from build123d import *

# Parameters (mm, degrees)
DODANIE_WYCI_GNI_CIE1_DEPTH = 5.325088567


with BuildPart() as part:
    # Szkic1 → Dodanie-wyciągnięcie1 (new body)
    with BuildSketch(Plane.XY):
        with BuildLine():
            Line((-0.951045555, 20.39370068), (-1.925922284, 17.39370068))
            ThreePointArc((-1.925922284, 17.39370068), (-2.737603138, 17.28454596), (-3.543288168, 17.13753509))
            Line((-3.543288168, 17.13753509), (-5.397502016, 19.689451162))
            ThreePointArc((-5.397502016, 19.689451162), (-6.515515156, 20.052693732), (-7.206498161, 19.101672684))
            Line((-7.206498161, 19.101672684), (-7.206610043, 15.947249659))
            ThreePointArc((-7.206610043, 15.947249659), (-7.944833745, 15.592614173), (-8.665656885, 15.203828161))
            Line((-8.665656885, 15.203828161), (-11.217704483, 17.05786098))
            ThreePointArc((-11.217704483, 17.05786098), (-12.393246293, 17.057840133), (-12.756528516, 15.939839877))
            Line((-12.756528516, 15.939839877), (-11.7818646, 12.93977073))
            ThreePointArc((-11.7818646, 12.93977073), (-12.374368671, 12.374368671), (-12.93977073, 11.7818646))
            Line((-12.93977073, 11.7818646), (-15.939839877, 12.756528516))
            ThreePointArc((-15.939839877, 12.756528516), (-17.057840133, 12.393246293), (-17.05786098, 11.217704483))
            Line((-17.05786098, 11.217704483), (-15.203828161, 8.665656885))
            ThreePointArc((-15.203828161, 8.665656885), (-15.592614173, 7.944833745), (-15.947249659, 7.206610043))
            Line((-15.947249659, 7.206610043), (-19.101672684, 7.206498161))
            ThreePointArc((-19.101672684, 7.206498161), (-20.052693732, 6.515515156), (-19.689451162, 5.397502016))
            Line((-19.689451162, 5.397502016), (-17.13753509, 3.543288168))
            ThreePointArc((-17.13753509, 3.543288168), (-17.28454596, 2.737603138), (-17.39370068, 1.925922284))
            Line((-17.39370068, 1.925922284), (-20.39370068, 0.951045555))
            ThreePointArc((-20.39370068, 0.951045555), (-21.084649954, 0), (-20.39370068, -0.951045555))
            Line((-20.39370068, -0.951045555), (-17.39370068, -1.925922284))
            ThreePointArc((-17.39370068, -1.925922284), (-17.28454596, -2.737603138), (-17.13753509, -3.543288168))
            Line((-17.13753509, -3.543288168), (-19.689451162, -5.397502016))
            ThreePointArc((-19.689451162, -5.397502016), (-20.052693732, -6.515515156), (-19.101672684, -7.206498161))
            Line((-19.101672684, -7.206498161), (-15.947249659, -7.206610043))
            ThreePointArc((-15.947249659, -7.206610043), (-15.592614173, -7.944833745), (-15.203828161, -8.665656885))
            Line((-15.203828161, -8.665656885), (-17.05786098, -11.217704483))
            ThreePointArc((-17.05786098, -11.217704483), (-17.057840133, -12.393246293), (-15.939839877, -12.756528516))
            Line((-15.939839877, -12.756528516), (-12.93977073, -11.7818646))
            ThreePointArc((-12.93977073, -11.7818646), (-12.374368671, -12.374368671), (-11.7818646, -12.93977073))
            Line((-11.7818646, -12.93977073), (-12.756528516, -15.939839877))
            ThreePointArc((-12.756528516, -15.939839877), (-12.393246293, -17.057840133), (-11.217704483, -17.05786098))
            Line((-11.217704483, -17.05786098), (-8.665656885, -15.203828161))
            ThreePointArc((-8.665656885, -15.203828161), (-7.944833745, -15.592614173), (-7.206610043, -15.947249659))
            Line((-7.206610043, -15.947249659), (-7.206498161, -19.101672684))
            ThreePointArc((-7.206498161, -19.101672684), (-6.515515156, -20.052693732), (-5.397502016, -19.689451162))
            Line((-5.397502016, -19.689451162), (-3.543288168, -17.13753509))
            ThreePointArc((-3.543288168, -17.13753509), (-2.737603138, -17.28454596), (-1.925922284, -17.39370068))
            Line((-1.925922284, -17.39370068), (-0.951045555, -20.39370068))
            ThreePointArc((-0.951045555, -20.39370068), (0, -21.084649954), (0.951045555, -20.39370068))
            Line((0.951045555, -20.39370068), (1.925922284, -17.39370068))
            ThreePointArc((1.925922284, -17.39370068), (2.737603138, -17.28454596), (3.543288168, -17.13753509))
            Line((3.543288168, -17.13753509), (5.397502016, -19.689451162))
            ThreePointArc((5.397502016, -19.689451162), (6.515515156, -20.052693732), (7.206498161, -19.101672684))
            Line((7.206498161, -19.101672684), (7.206610043, -15.947249659))
            ThreePointArc((7.206610043, -15.947249659), (7.944833745, -15.592614173), (8.665656885, -15.203828161))
            Line((8.665656885, -15.203828161), (11.217704483, -17.05786098))
            ThreePointArc((11.217704483, -17.05786098), (12.393246293, -17.057840133), (12.756528516, -15.939839877))
            Line((12.756528516, -15.939839877), (11.7818646, -12.93977073))
            ThreePointArc((11.7818646, -12.93977073), (12.374368671, -12.374368671), (12.93977073, -11.7818646))
            Line((12.93977073, -11.7818646), (15.939839877, -12.756528516))
            ThreePointArc((15.939839877, -12.756528516), (17.057840133, -12.393246293), (17.05786098, -11.217704483))
            Line((17.05786098, -11.217704483), (15.203828161, -8.665656885))
            ThreePointArc((15.203828161, -8.665656885), (15.592614173, -7.944833745), (15.947249659, -7.206610043))
            Line((15.947249659, -7.206610043), (19.101672684, -7.206498161))
            ThreePointArc((19.101672684, -7.206498161), (20.052693732, -6.515515156), (19.689451162, -5.397502016))
            Line((19.689451162, -5.397502016), (17.13753509, -3.543288168))
            ThreePointArc((17.13753509, -3.543288168), (17.28454596, -2.737603138), (17.39370068, -1.925922284))
            Line((17.39370068, -1.925922284), (20.39370068, -0.951045555))
            ThreePointArc((20.39370068, -0.951045555), (21.084649954, 0), (20.39370068, 0.951045555))
            Line((20.39370068, 0.951045555), (17.39370068, 1.925922284))
            ThreePointArc((17.39370068, 1.925922284), (17.28454596, 2.737603138), (17.13753509, 3.543288168))
            Line((17.13753509, 3.543288168), (19.689451162, 5.397502016))
            ThreePointArc((19.689451162, 5.397502016), (20.052693732, 6.515515156), (19.101672684, 7.206498161))
            Line((19.101672684, 7.206498161), (15.947249659, 7.206610043))
            ThreePointArc((15.947249659, 7.206610043), (15.592614173, 7.944833745), (15.203828161, 8.665656885))
            Line((15.203828161, 8.665656885), (17.05786098, 11.217704483))
            ThreePointArc((17.05786098, 11.217704483), (17.057840133, 12.393246293), (15.939839877, 12.756528516))
            Line((15.939839877, 12.756528516), (12.93977073, 11.7818646))
            ThreePointArc((12.93977073, 11.7818646), (12.374368671, 12.374368671), (11.7818646, 12.93977073))
            Line((11.7818646, 12.93977073), (12.756528516, 15.939839877))
            ThreePointArc((12.756528516, 15.939839877), (12.393246293, 17.057840133), (11.217704483, 17.05786098))
            Line((11.217704483, 17.05786098), (8.665656885, 15.203828161))
            ThreePointArc((8.665656885, 15.203828161), (7.944833745, 15.592614173), (7.206610043, 15.947249659))
            Line((7.206610043, 15.947249659), (7.206498161, 19.101672684))
            ThreePointArc((7.206498161, 19.101672684), (6.515515156, 20.052693732), (5.397502016, 19.689451162))
            Line((5.397502016, 19.689451162), (3.543288168, 17.13753509))
            ThreePointArc((3.543288168, 17.13753509), (2.737603138, 17.28454596), (1.925922284, 17.39370068))
            Line((1.925922284, 17.39370068), (0.951045555, 20.39370068))
            ThreePointArc((0.951045555, 20.39370068), (0, 21.084649954), (-0.951045555, 20.39370068))
        make_face()
        with BuildLine():
            Line((-2, 1.5), (-2, -1.5))
            ThreePointArc((-2, -1.5), (2.5, 0), (-2, 1.5))
        make_face(mode=Mode.SUBTRACT)
    extrude(amount=DODANIE_WYCI_GNI_CIE1_DEPTH)


solid = part.part
CAD build for the part. Positions are in the model's coordinates, mm. A direction names the side the tool comes from. Coordinates: 2 decimals unless noted, no trailing zeros. Write each loop counter-clockwise with the first axis right and the second up, starting at its lowest first coordinate (ties: lowest second). Pieces come first, ordered by that corner, then holes. Notation, with made-up numbers: (3, 87) - (29, 87) arc R20 ccw to (29, 126) - close; hole circle Ø1 at (45, 34.5). An arc over 180 degrees is marked (long way). Use a Markdown table: item, result. Add a question column.
Item 1: Band-saw the part on B-B, the plane y = 0. Give the cut face in (x, z), and give its area (3 significant figures).
Item 2: Band-saw the part on A-A, the plane x = 0. Give the cut face in (y, z), and give its area (3 significant figures).
Item 3: Band-saw the part on D-D, the plane x = -13.5. Give the cut face in (y, z), and give its area (3 significant figures).
Item 4: Drill centre lines: L1, parallel to X at y = 19.5, z = 2.1; L2, parallel to Y at x = -16, z = 3.35; L3, parallel to X at y = 3, z = 1.4. Where is each one in solid material? Low to high. Write a range as from..to.
Item 5: 3-axis set-ups, long thin cutter, end or side, ignore diameter. For faces 1 (the face through (18.915, 1.432, 2.625)), 2 (the face through (-16.1, -9.9, 2.6)), 3 (the face through (-12.38, -12.37, 2.63)), 4 (the face through (9.9, -16.1, 2.6)), 5 (the face through (-14.419, 12.262, 2.625)): which of +Z, -Z, +X, -X, +Y, -Y reach the whole face in a straight line?
Item 6: Band-saw the part on C-C, the plane y = 4.5. Give the cut face in (x, z).
Item 7: Flat gauge pins, fed straight in: pin 1 (1.6 mm diameter, centred on x = -17, z = 2.5, fed in from -Y); pin 2 (2.5 mm diameter, centred on y = -17, z = 2, fed in from -X); pin 3 (2.5 mm diameter, centred on y = -17.5, z = 2.5, fed in from +X). Where does each tip first touch, or does it go through?
Item 8: Mould opens along Y. For faces 6 (the face through (-16.144, 9.96, 2.625)), 7 (the face through (7.93, -15.6, 2.63)), 8 (the face through (4.48, 18.43, 2.63)) say: pulls with the +Y half, pulls with the -Y half, needs draft (parallel to the pull), parting line crosses it, or undercut.
Numbers:
| question | item | result |
|---|---|---|
| 1 | outline | (-21.08, 0) - (-2, 0) - (-2, 5.33) - (-21.08, 5.33) - close; (2.5, 0) - (21.08, 0) - (21.08, 5.33) - (2.5, 5.33) - close |
| 1 | area | 201 mm2 |
| 2 | outline | (-21.08, 0) - (-2.5, 0) - (-2.5, 5.33) - (-21.08, 5.33) - close; (2.5, 0) - (21.08, 0) - (21.08, 5.33) - (2.5, 5.33) - close |
| 2 | area | 198 mm2 |
| 3 | outline | (-11.96, 0) - (11.96, 0) - (11.96, 5.33) - (-11.96, 5.33) - close |
| 3 | area | 127 mm2 |
| 4 | L1 | -7.12..-5.26, -1.24..1.24, 5.26..7.12 |
| 4 | L2 | -12.77..-9.76, -7.21..7.21, 9.76..12.77 |
| 4 | L3 | -17.24..17.24 |
| 5 | face 1 | +Z, -Z, +X |
| 5 | face 2 | +Z, -Z, -X |
| 5 | face 3 | +Z, -Z |
| 5 | face 4 | +Z, -Z, -Y |
| 5 | face 5 | +Z, -Z, +Y |
| 6 | outline | (-18.45, 0) - (18.45, 0) - (18.45, 5.33) - (-18.45, 5.33) - close |
| 7 | pin 1 | y = -12.81 |
| 7 | pin 2 | x = -12.81 |
| 7 | pin 3 | x = 12.81 |
| 8 | face 6 | undercut |
| 8 | face 7 | pulls with the -Y half |
| 8 | face 8 | pulls with the +Y half |
